Design review of the part built by this model. Coordinates are the model's own, in mm. Face numbers are marked on the shaded views. A direction names the side the tool comes from. Coordinates: 2 decimals unless noted, no trailing zeros. Order: outer loops, then holes, each group sorted by start corner. A loop starts at its lowest first (then second) coordinate and runs counter-clockwise, first axis right, second up. Notation, with made-up numbers: M 73,-7.5 L 84,-7.5 A28 ccw 84,25.5 Z; hole C 45,-23.75 d3. An arc over 180 degrees is marked long. Answer in a Markdown table with one row per item.
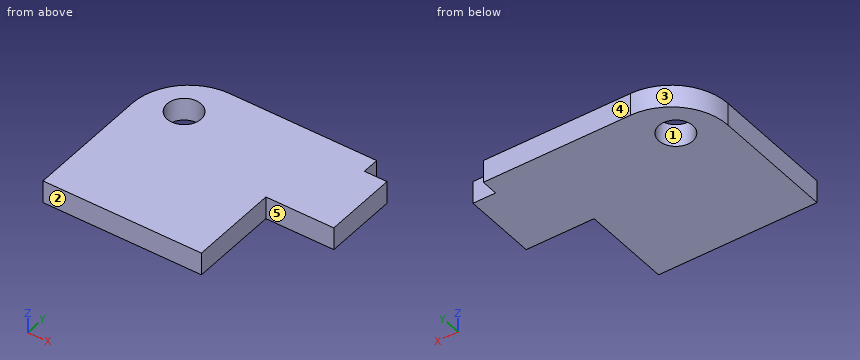
from build123d import *

# Parameters (mm, degrees)
SKETCH1_R           = 1.5
BOSS_EXTRUDE1_DEPTH = 2


with BuildPart() as part:
    # Sketch1 → Boss-Extrude1 (new body)
    with BuildSketch(Plane.XY):
        with BuildLine():
            Line((14, -8), (20, -8))
            Line((20, -8), (20, -1.5))
            Line((20, -1.5), (18, -1.5))
            Line((18, -1.5), (18, 0))
            Line((18, 0), (5, 0))
            ThreePointArc((5, 0), (1.464466094, -1.464466094), (0, -5))
            Line((0, -5), (0, -15.875626598))
            Line((0, -15.875626598), (14, -15.875626598))
            Line((14, -15.875626598), (14, -8))
        make_face()
        with Locations((3.560660172, -3.560660172)):
            Circle(SKETCH1_R, mode=Mode.SUBTRACT)
    extrude(amount=BOSS_EXTRUDE1_DEPTH)


solid = part.part
(1) For the marked faces 4 and 5, list the 3-axis set-ups (+Z, -Z, +X, -X, +Y, -Y) from which the entire face can be reached by the end or side of a thin tool; tool diameter is ignored.
Return value:
| item | result |
|---|---|
| face 4 | +Z, -Z, +X, -X, +Y |
| face 5 | +Z, -Z, +X, -Y |
(2) Add section D-D, the plane x = 16.25. Give the boundary of the cut face in (y, z), and give its area (3 significant figures).
Return value:
| item | result |
|---|---|
| outline | M -8,0 L 0,0 L 0,2 L -8,2 Z |
| area | 16.0 mm2 |
(3) Add section C-C, the plane z = 0.5. Give the boundary of the cut face in (x, y), and give its area (3 significant figures).
Return value:
| item | result |
|---|---|
| outline | M 0,-15.88 L 14,-15.88 L 14,-8 L 20,-8 L 20,-1.5 L 18,-1.5 L 18,0 L 5,0 A5 ccw 0,-5 Z; hole C 3.56,-3.56 d3 |
| area | 255 mm2 |
(4) Insertion check: pin 1 Ø1.2 at (y, z) = (-0.5, 0.5) entering from +X; pin 2 Ø1 at (x, z) = (19, 1) entering from +Y. Each pin has a flat end and moves straight along its axis. Give the tip position at first contact, or say it passes through.
Return value:
| item | result |
|---|---|
| pin 1 | stops at x = 18 |
| pin 2 | stops at y = -1.5 |
(5) Add section B-B, the plane y = -4.25. Give the boundary of the cut face in (x, z).
Return value:
| item | result |
|---|---|
| outline | M 0.06,0 L 2.23,0 L 2.23,2 L 0.06,2 Z; M 4.89,0 L 20,0 L 20,2 L 4.89,2 Z |
(6) Add section A-A, the plane x = 3.75. Give the boundary of the cut face in (y, z), and give its area (3 significant figures).
Return value:
| item | result |
|---|---|
| outline | M -15.88,0 L -5.05,0 L -5.05,2 L -15.88,2 Z; M -2.07,0 L -0.16,0 L -0.16,2 L -2.07,2 Z |
| area | 25.5 mm2 |
(7) For line 1 along X through (y, z) = (-14.75, 1.8); line 2 along Y through (x, z) = (14.5, 0.75); line 3 along Y through (x, z) = (3.25, 1.5), list the stretches that pass through material, from the lowest coordinate up. Write a range as from..to.
Return value:
| item | result |
|---|---|
| line 1 | x = 0..14 |
| line 2 | y = -8..0 |
| line 3 | y = -15.88..-5.03, -2.09..-0.32 |
(8) Draft analysis for pull direction Y (two halves, no side actions). For the marked faces 1, 2 and 3, state which applies: pulls with the +Y half, pulls with the -Y half, needs draft (parallel to the pull), parting line crosses it, or undercut.
Return value:
| item | result |
|---|---|
| face 1 | undercut |
| face 2 | pulls with the -Y half |
| face 3 | pulls with the +Y half |
